The listing builds one solid part. Answer for the finished solid, in the listing's coordinates (mm). Round coordinates to 2 decimals unless told otherwise and drop trailing zeros. Write each loop counter-clockwise with the first axis right and the second up, starting at its lowest first coordinate (ties: lowest second). Pieces come first, ordered by that corner, then holes. Notation, with made-up numbers: (-33.5, 27.25) -> (0.5, 27.25) arc R27 ccw to (0.5, 66.25) -> close; hole circle Ø7 at (83.25, -11). An arc over 180 degrees is marked (long way). Write each question's results on one line, items separated by ' | '. Start each with the question number.
```python
from build123d import *

# Parameters (mm, degrees)
F0_W      = 84
F0_H      = 21
F0_W_2    = 78
F0_H_2    = 3
F0_W_3    = 72
F0_R      = 1.5
F1_DEPTH  = 2
F2_W      = 2
F2_H      = 21
F3_DEPTH  = 5
F4_W      = 2
F4_H      = 21
F5_DEPTH  = 5
F6_R      = 1.5
F7_DEPTH  = 25
F8_R      = 1
F9_W      = 1
F9_H      = 21
F10_DEPTH = 25


with BuildPart() as f1:
    # F0 (on Front) → F1 (new body)
    with BuildSketch(Plane.XZ):
        Rectangle(F0_W, F0_H)
        with Locations((0, -6)):
            Rectangle(F0_W_2, F0_H_2, mode=Mode.SUBTRACT)
        with Locations((-3, 6)):
            Rectangle(F0_W_3, F0_H_2, mode=Mode.SUBTRACT)
        Rectangle(F0_W_2, F0_H_2, mode=Mode.SUBTRACT)
        with Locations((37.5, 6)):
            Circle(F0_R, mode=Mode.SUBTRACT)
    extrude(amount=F1_DEPTH)

    # F2 (on face) → F3 (join)
    with BuildSketch(Plane.YZ.offset(42)):
        with Locations((-1, 0)):
            Rectangle(F2_W, F2_H)
    extrude(amount=F3_DEPTH)

    # F4 (on face) → F5 (join)
    with BuildSketch(Plane(origin=(-42, 0, 0), x_dir=(0, -1, 0), z_dir=(-1, 0, 0))):
        with Locations((1, 0)):
            Rectangle(F4_W, F4_H)
    extrude(amount=F5_DEPTH)

    # F6 (on face) → F7 (cut)
    with BuildSketch(Plane.XZ.offset(2)):
        with Locations((-42.5, 6)):
            Circle(F6_R)
        with Locations((-42.5, -6)):
            Circle(F6_R)
        with Locations((42.5, 6)):
            Circle(F6_R)
        with Locations((42.5, -6)):
            Circle(F6_R)
    extrude(amount=-F7_DEPTH, mode=Mode.SUBTRACT)

    # F8
    f8_edges = [f1.edges().sort_by_distance(p)[0] for p in [
        (-39, -1, 7.5),
        (-39, -1, 1.5),
        (-39, -1, -4.5),
        (-39, -1, 4.5),
        (-39, -1, -1.5),
        (-39, -1, -7.5),
        (33, -1, 7.5),
        (39, -1, 1.5),
        (39, -1, -4.5),
        (39, -1, -7.5),
        (39, -1, -1.5),
        (33, -1, 4.5),
    ]]
    fillet(f8_edges, radius=F8_R)

    # F9 (on face) → F10 (cut)
    with BuildSketch(Plane.XZ.offset(2)):
        with Locations((-46.5, 0)):
            Rectangle(F9_W, F9_H)
        with Locations((46.5, 0)):
            Rectangle(F9_W, F9_H)
    extrude(amount=-F10_DEPTH, mode=Mode.SUBTRACT)


solid = f1.part
```
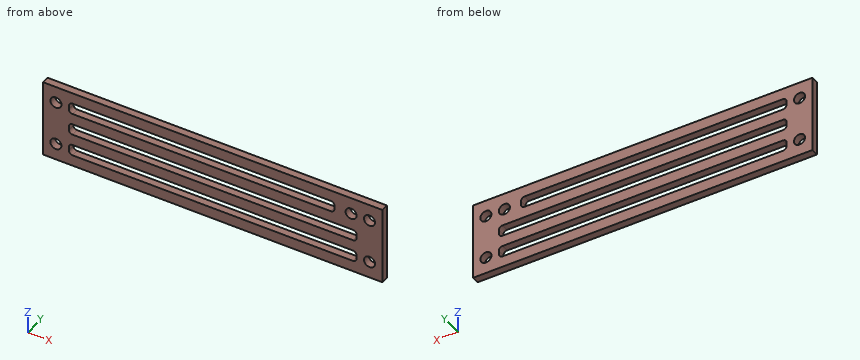
Q1. The part is cut by section A-A, the plane x = 42.5. Write down the section's boundary in (y, z).
Q2. Find the intervals of material crossed by line 1 (Z direction, x = -16, y = -0.4); line 2 (Z direction, x = -42.5, y = -0.65); line 3 (X direction, y = -0.3, z = -0.5), in increasing order.
Q3. The part is cut by section C-C, the plane x = 28. Write down the section's boundary in (y, z), then the cut area to 3 significant figures.
Q4. The part is cut by section B-B, the plane y = -1.2. State how many separate pieces and enclosed holes the cut face has, then the cut area to 3 significant figures.
Q5. This flat-tipped pin is pushed along its axis until it touches: pin 1 (1.8 mm diameter, centred on x = -42.5, z = 6, fed in from -Y). Where does it stop, or does it pass through?
Answers follow:
1) outline: (-2, -10.5) -> (0, -10.5) -> (0, -7.5) -> (-2, -7.5) -> close; (-2, -4.5) -> (0, -4.5) -> (0, 4.5) -> (-2, 4.5) -> close; (-2, 7.5) -> (0, 7.5) -> (0, 10.5) -> (-2, 10.5) -> close
2) line 1: -10.5 to -7.5, -4.5 to -1.5, 1.5 to 4.5, 7.5 to 10.5 | line 2: -10.5 to -7.5, -4.5 to 4.5, 7.5 to 10.5 | line 3: -46 to -39, 39 to 46
3) outline: (-2, -10.5) -> (0, -10.5) -> (0, -7.5) -> (-2, -7.5) -> close; (-2, -4.5) -> (0, -4.5) -> (0, -1.5) -> (-2, -1.5) -> close; (-2, 1.5) -> (0, 1.5) -> (0, 4.5) -> (-2, 4.5) -> close; (-2, 7.5) -> (0, 7.5) -> (0, 10.5) -> (-2, 10.5) -> close | area: 24.0 mm^2
4) separate pieces: 1 | enclosed holes: 8 | area: 1,220 mm^2
5) pin 1: through
